Source: CAD feature listing. Evaluate the final solid. Frame: model axes, mm. Face numbers are marked on the shaded views. Give positions to 0.01 mm unless a question says otherwise; leave off trailing zeros. Order: outer loops, then holes, each group sorted by start corner. A loop starts at its lowest first (then second) coordinate and runs counter-clockwise, first axis right, second up. Notation, with made-up numbers: M 49.5,68 L 92.5,68 A17 cw 92.5,72 Z; hole C 44.25,-19 d8. An arc over 180 degrees is marked long. Answer in a Markdown table with one row per item. Add a question column.
(1) Section query B-B, the plane y = 33.5. Return loops of the section in (x, z), plus the area to 3 significant figures.
(2) Pin query (flat end, axial travel): P1, Ø3, axis at x = 12.06, y = 36.57, coming from the -Z side. Return the tip coordinate at first contact, or that it passes through.
(3) Section query A-A, the plane x = 9.5. Return loops of the section in (y, z), plus the area to 3 significant figures.
(4) Mould query, pull axis Y, two halves, no side actions, for the marked faces 1 and 2. Classes: pulls with the +Y half, pulls with the -Y half, needs draft (parallel to the pull), parting line crosses it, or undercut.
(5) Section query C-C, the plane x = 18. Return loops of the section in (y, z), plus the area to 3 significant figures.
(6) Section query D-D, the plane z = 0.9. Count the separate pieces of the cut face and the enclosed holes in it, plus the area to 3 significant figures.
(7) Material intervals for line 1 along X through (y, z) = (4, 1.25); line 2 along X through (y, z) = (33, 1.3); line 3 along Y through (x, z) = (4.25, 0.6), sorted ascending.
Autodesk Inventor part; units mm, degrees
ref_plane "YZ Plane" through (0, 0, 0) normal (1, 0, 0) x (0, 1, 0)
ref_plane "XZ Plane" through (0, 0, 0) normal (0, 1, 0) x (-1, 0, 0)
ref_plane "XY Plane" through (0, 0, 0) normal (0, 0, 1) x (1, 0, 0)
sketch "Sketch1" plane through (0, 0, 0) normal (0, 0, 1) x (1, 0, 0)
  line L0 (0, 0) -> (24.13, 0)
  line L1 (24.13, 0) -> (24.13, 39.116)
  line L2 (24.13, 39.116) -> (0, 39.116)
  line L3 (0, 39.116) -> (0, 0)
  dimension "d0" = 39.116
  dimension "d1" = 24.13
extrude "Extrusion1" add sketch "Sketch1" along normal blind 2.54
sketch "Sketch3" plane through (0, 0, 0) normal (0, -1, 0) x (1, 0, 0)
  circle A0 centre (3.9772, 1.2808) radius 0.9652
  circle A1 centre (20.3157, 1.2808) radius 0.9652
  point P0 (0, 0)
  dimension "d7" = 1.9304
  dimension "d8" = 1.9304
hole "Hole1" at (3.9772, 0, 1.2808) at (20.3157, 0, 1.2808) direction (0, 1, 0) diameter 1.6942 depth 5.7785 tip angle 118
sketch "Sketch5" plane through (0, 0, 2.54) normal (0, 0, 1) x (1, 0, 0)
  circle A0 centre (12.065, 28.5714) radius 3.4925
  circle A1 centre (12.065, 28.5714) radius 8.001
  circle A2 centre (18.9941, 32.5719) radius 1.5875
  circle A3 centre (12.065, 36.5724) radius 1.5875
  circle A4 centre (12.065, 28.5714) radius 8.001
  circle A5 centre (5.1359, 32.5719) radius 1.5875
  circle A6 centre (12.065, 28.5714) radius 8.001
  circle A7 centre (5.1359, 24.5709) radius 1.5875
  circle A8 centre (12.065, 28.5714) radius 8.001
  circle A9 centre (12.065, 20.5704) radius 1.5875
  circle A10 centre (12.065, 28.5714) radius 8.001
  circle A11 centre (18.9941, 24.5709) radius 1.5875
  circle A12 centre (12.065, 28.5714) radius 8.001
  line L0 (24.13, 0) -> (24.13, 39.116)
  line L1 (24.13, 39.116) -> (0, 39.116)
  line L2 (0, 0) -> (24.13, 0)
  line L3 (12.065, 39.116) -> (12.065, 28.5714)
  dimension "d32" = 16.002
  dimension "d31" = 6.985
  dimension "d33" = 3.175
  dimension "d34" = 360
  dimension "d35" = 24.13
extrude "Extrusion4" cut sketch "Sketch5" against normal through all contours A0 | A3 A1 L3 | L3 A1 A3 | A3 L3 A1 | A1 L3 A3 | A5 A1 | A1 A5 | A2 A1 | A1 A2 | A7 A1 | A1 A7 | A11 A1 | A1 A11 | A9 A1 | A1 A9
properties part number "collection motor mount"
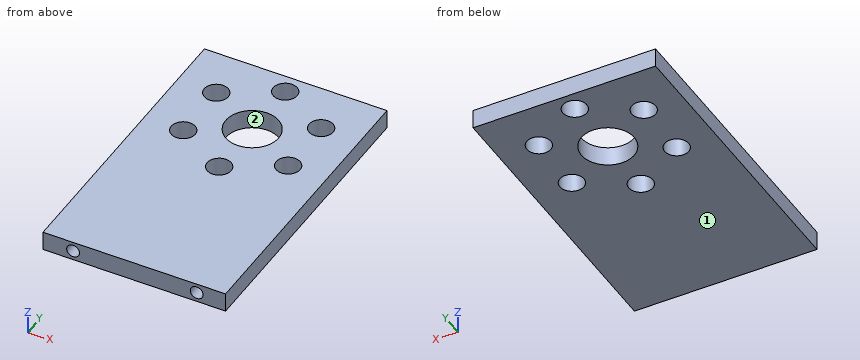
Values follow:
| question | item | result |
|---|---|---|
| 1 | outline | M 0,0 L 3.85,0 L 3.85,2.54 L 0,2.54 Z; M 6.42,0 L 17.71,0 L 17.71,2.54 L 6.42,2.54 Z; M 20.28,0 L 24.13,0 L 24.13,2.54 L 20.28,2.54 Z |
| 1 | area | 48.2 mm² |
| 2 | P1 | passes through |
| 3 | outline | M 0,0 L 26.2,0 L 26.2,2.54 L 0,2.54 Z; M 30.94,0 L 39.12,0 L 39.12,2.54 L 30.94,2.54 Z |
| 3 | area | 87.3 mm² |
| 4 | face 1 | needs draft |
| 4 | face 2 | undercut |
| 5 | outline | M 0,0 L 23.33,0 L 23.33,2.54 L 0,2.54 Z; M 25.81,0 L 31.33,0 L 31.33,2.54 L 25.81,2.54 Z; M 33.81,0 L 39.12,0 L 39.12,2.54 L 33.81,2.54 Z |
| 5 | area | 86.8 mm² |
| 6 | separate pieces | 1 |
| 6 | enclosed holes | 7 |
| 6 | area | 840 mm² |
| 7 | line 1 | x = 0 to 3.13, 4.82 to 19.47, 21.16 to 24.13 |
| 7 | line 2 | x = 0 to 3.61, 6.66 to 17.47, 20.52 to 24.13 |
| 7 | line 3 | y = 5.85 to 23.25, 25.89 to 31.25, 33.89 to 39.12 |
